For this review, take the finished solid that the model builds, in its own axes (mm). A direction names the side the tool comes from. Round coordinates to 2 decimals unless told otherwise and drop trailing zeros. Loops run counter-clockwise (first coordinate to the right, second up) from the corner with the lowest first, then second, coordinate; pieces in that order, holes last. Notation, with made-up numbers: M -19.5,32 L 13.5,32 A11 ccw 13.5,47 Z; hole C -19,64.5 d1. An arc over 180 degrees is marked long. One line per question, with ' | ' between items. Start each with the question number.
1) We need section B-B (y = 4). Give the boundary of the cut face in (x, z) (3 decimals).
2) We need section C-C (y = 7). Give the boundary of the cut face in (x, z) (3 decimals), and give its area (3 significant figures).
3) For faces 1 (the face through (5.4, 14, 1)), 2 (the face through (-2.738, 14.712, 4.655)), 3 (the face through (-2.66, 14.71, -4.7)), 4 (the face through (0, 12, 0)), list the 3-axis set-ups (+Z, -Z, +X, -X, +Y, -Y) from which the entire face can be reached by the end or side of a thin tool; tool diameter is ignored.
4) We need section D-D (x = -1.5). Give the boundary of the cut face in (y, z).
5) Mouldability with a two-part tool opening along X and no side actions: class faces 5 (the face through (0.94, 5.92, -2.98)), 6 (the face through (0, 17.5, 0)), 7 (the face through (-8, 6, 0)) as pulls with the +X half, pulls with the -X half, needs draft (parallel to the pull), parting line crosses it, or undercut.
6) For pin 1 Ø3 at (y, z) = (14.5, 1) entering from -X; pin 2 Ø2 at (x, z) = (2.5, 7) entering from +Y; pin 3 Ø4 at (x, y) = (3.5, 3.5) entering from +Z, all flat-tipped, find the tip position at first contact; note any pin that passes through.
7) For probe 1 along Y at (x, z) = (5, 0); probe 2 along Y at (x, z) = (-0.75, 0); probe 3 along X at (y, z) = (6.5, 0) (3 decimals), list the stretches that pass through material, from the lowest coordinate up. Write a range as from..to.
8) We need section A-A (z = 0). Give the boundary of the cut face in (x, y) (3 decimals), and give its area (3 significant figures).
```python
from build123d import *

# Parameters (mm, degrees)
ESBO_O1_R                = 9
RESSALTO_EXTRUS_O1_DEPTH = 12
RESSALTO_EXTRUS_O2_DEPTH = 5.5
ESBO_O3_R                = 1
CORTE_EXTRUS_O1_DEPTH    = 25.384626304
ESBO_O4_R                = 3.125
CORTE_EXTRUS_O2_DEPTH    = 12
CORTE_EXTRUS_O3_REACH    = 23.639
ESBO_O6_R                = 1.25
CORTE_EXTRUS_O4_DEPTH    = 26.362373706


with BuildPart() as part:
    # Esboço1 → Ressalto-extrusão1 (new body)
    with BuildSketch(Plane(origin=(0, 0, 0), x_dir=(1, 0, 0), z_dir=(0, 1, 0))):
        with Locations(Location((0, 0, 0), (0, 0, 270))):
            Circle(ESBO_O1_R)
    extrude(amount=RESSALTO_EXTRUS_O1_DEPTH)

    # Esboço2 → Ressalto-extrusão2 (add)
    with BuildSketch(Plane(origin=(0, 12, 0), x_dir=(1, 0, 0), z_dir=(0, 1, 0))):
        Polygon((0, 6.235382907), (-5.4, 3.117691454), (-5.4, -3.117691454), (0, -6.235382907), (5.4, -3.117691454), (5.4, 3.117691454), align=None)
    extrude(amount=RESSALTO_EXTRUS_O2_DEPTH)

    # Esboço3 → Corte-extrusão1 (cut, through all)
    with BuildSketch(Plane.ZY.offset(5.4)):
        with Locations((0, 15)):
            Circle(ESBO_O3_R)
    extrude(amount=-CORTE_EXTRUS_O1_DEPTH, mode=Mode.SUBTRACT)

    # Esboço4 → Corte-extrusão2 (cut)
    with BuildSketch(Plane.XZ):
        with Locations(Location((0, 0, 0), (0, 0, 270))):
            Circle(ESBO_O4_R)
    extrude(amount=-CORTE_EXTRUS_O2_DEPTH, mode=Mode.SUBTRACT)

    # Esboço5 → Corte-extrusão3 (cut, up to next)
    with BuildSketch(Plane.XZ, mode=Mode.PRIVATE) as corte_extrus_o3_sk1:
        with BuildLine():
            Line((-8, -4.123105626), (-8, 4.123105626))
            ThreePointArc((-8, 4.123105626), (-9, 0), (-8, -4.123105626))
        make_face()
    corte_extrus_o3_tool1 = extrude(corte_extrus_o3_sk1.sketch, amount=-CORTE_EXTRUS_O3_REACH, mode=Mode.PRIVATE) & part.part
    # Esboço5 → Corte-extrusão3 (cut, up to next)
    with BuildSketch(Plane.XZ, mode=Mode.PRIVATE) as corte_extrus_o3_sk2:
        with BuildLine():
            Line((8, -4.123105626), (8, 4.123105626))
            ThreePointArc((8, 4.123105626), (9, 0), (8, -4.123105626))
        make_face()
    corte_extrus_o3_tool2 = extrude(corte_extrus_o3_sk2.sketch, amount=-CORTE_EXTRUS_O3_REACH, mode=Mode.PRIVATE) & part.part
    add(corte_extrus_o3_tool1.solids().sort_by_distance((-8.401968, 0, 0))[0], mode=Mode.SUBTRACT)
    add(corte_extrus_o3_tool2.solids().sort_by_distance((8.401968, 0, 0))[0], mode=Mode.SUBTRACT)

    # Esboço6 → Corte-extrusão4 (cut, through all)
    with BuildSketch(Plane.ZY.offset(8)):
        with Locations((0, 4)):
            Circle(ESBO_O6_R)
    extrude(amount=-CORTE_EXTRUS_O4_DEPTH, mode=Mode.SUBTRACT)


solid = part.part
```
Answers below:
1) outline: M -8,-4.123 A9 ccw 8,-4.123 L 8,-1.25 L 2.864,-1.25 A3.125 cw -2.864,-1.25 L -8,-1.25 Z; M -8,1.25 L -2.864,1.25 A3.125 cw 2.864,1.25 L 8,1.25 L 8,4.123 A9 ccw -8,4.123 Z
2) outline: M -8,-4.123 A9 ccw 8,-4.123 L 8,4.123 A9 ccw -8,4.123 Z; hole C 0,0 d6.25 | area: 213 mm^2
3) face 1: +Z, -Z, +X, +Y | face 2: +Z, -X, +Y | face 3: -Z, -X, +Y | face 4: -Y
4) outline: M 0,-8.87 L 12,-8.87 L 12,-5.37 L 17.5,-5.37 L 17.5,5.37 L 12,5.37 L 12,8.87 L 0,8.87 L 0,2.74 L 12,2.74 L 12,-2.74 L 0,-2.74 Z; hole C 15,0 d2
5) face 5: undercut | face 6: needs draft | face 7: pulls with the -X half
6) pin 1: x = -5.4 | pin 2: y = 12 | pin 3: z = 8.87
7) probe 1: 0..2.75, 5.25..14, 16..17.5 | probe 2: 12..14, 16..17.5 | probe 3: -8..-3.125, 3.125..8
8) outline: M -8,0 L -3.125,0 L -3.125,2.75 L -8,2.75 Z; M -8,5.25 L -3.125,5.25 L -3.125,12 L 3.125,12 L 3.125,5.25 L 8,5.25 L 8,12 L 5.4,12 L 5.4,14 L -5.4,14 L -5.4,12 L -8,12 Z; M -5.4,16 L 5.4,16 L 5.4,17.5 L -5.4,17.5 Z; M 3.125,0 L 8,0 L 8,2.75 L 3.125,2.75 Z | area: 130 mm^2
